```python
from build123d import *

# Parameters (mm, degrees)
BOSS_EXTRUDE2_DEPTH = 10
CUT_EXTRUDE9_DEPTH  = 3
BOSS_EXTRUDE3_DEPTH = 25
CUT_EXTRUDE11_DEPTH = 15


with BuildPart() as part:
    # Sketch1 → Boss-Extrude2 (new body)
    with BuildSketch(Plane(origin=(0, 0, 0), x_dir=(0, 0, -1), z_dir=(1, 0, 0))):
        Polygon((0, 0), (2, 0), (2, 9.1), (6.2, 13.3), (30, 13.3), (30, 15.3), (0, 15.3), align=None)
    extrude(amount=BOSS_EXTRUDE2_DEPTH)

    # Sketch2 → Cut-Extrude9 (cut)
    with BuildSketch(Plane(origin=(0, 15.3, 0), x_dir=(1, 0, 0), z_dir=(0, 1, 0))):
        with BuildLine():
            ThreePointArc((7, 15), (5, 17), (3, 15))
            Line((3, 15), (7, 15))
        make_face()
        with BuildLine():
            Line((7, 15), (3, 15))
            ThreePointArc((3, 15), (5, 13), (7, 15))
        make_face()
    extrude(amount=-CUT_EXTRUDE9_DEPTH, mode=Mode.SUBTRACT)

    # Sketch1<14> → Boss-Extrude3 (add)
    with BuildSketch(Plane(origin=(0, 0, 0), x_dir=(0, 0, -1), z_dir=(1, 0, 0))):
        Polygon((0, 7.6), (0, 0), (2, 0), (2, 9.1), (6.2, 13.3), (6.2, 15.3), (0, 15.3), (0, 12.4), (-1.8, 12.4), (-1.8, 15.25), (-4.55, 12.5), (-4.55, 7.671680622), (-1.8, 4.921680622), (-1.8, 7.6), align=None)
    extrude(amount=-BOSS_EXTRUDE3_DEPTH)

    # Sketch1<18> → Cut-Extrude11 (cut)
    with BuildSketch(Plane(origin=(0, 0, 0), x_dir=(0, 0, -1), z_dir=(1, 0, 0))):
        Polygon((-1.8, 7.6), (0, 7.6), (0, 12.4), (-1.8, 12.4), (-1.8, 15.25), (-4.55, 12.5), (-4.55, 7.671680622), (-1.8, 4.921680622), align=None)
    extrude(amount=-CUT_EXTRUDE11_DEPTH, mode=Mode.SUBTRACT)


solid = part.part
```
Input: part model. Units: mm. Frame: model coordinates. A direction names the side the tool comes from. Coordinates: 2 decimals unless noted, no trailing zeros. Loops run counter-clockwise (first coordinate to the right, second up) from the corner with the lowest first, then second, coordinate; pieces in that order, holes last. Notation, with made-up numbers: M 52,15.5 L 107,15.5 A7 ccw 107,24.5 Z; hole C 23.25,83 d5. An arc over 180 degrees is marked long. Answer in a Markdown table with one row per item.
1. Material intervals for line 1 (Z direction, x = 5, y = 14.05); line 2 (Z direction, x = -11.5, y = 6); line 3 (Z direction, x = -19.5, y = 6.25), sorted ascending.
Response:
| item | result |
|---|---|
| line 1 | z = -30 to -17, -13 to 0 |
| line 2 | z = -2 to 0 |
| line 3 | z = -2 to 0, 1.8 to 3.13 |
2. Draft query along Z for faces 1 (the flat face through (-12, 14, -6.2)), 2 (the flat face through (5, 13.3, -18)), 3 (the flat face through (-20, 12.4, 1)). Return one class per face: pulls with the +Z half, pulls with the -Z half, needs draft (parallel to the pull), parting line crosses it, or undercut.
Response:
| item | result |
|---|---|
| face 1 | pulls with the -Z half |
| face 2 | needs draft |
| face 3 | undercut |
3. First-contact query: pin 1 (3 mm diameter, centred on x = 5, z = -15, fed in from -Y); pin 2 (1.4 mm diameter, centred on x = -21, y = 13.5, fed in from -Z); pin 3 (4.5 mm diameter, centred on x = -16, y = 3, fed in from -Z); pin 4 (5 mm diameter, centred on x = -4.5, y = 4.5, fed in from +Z). Flat tips, straight axial feed; report the tip coordinate or a pass-through.
Response:
| item | result |
|---|---|
| pin 1 | passes through |
| pin 2 | stops at z = -6.2 |
| pin 3 | stops at z = -2 |
| pin 4 | stops at z = 0 |
4. Section C-C, the plane x = -5. Output: boundary loops of the cut face in (y, z), then the cut area to 3 significant figures.
Response:
| item | result |
|---|---|
| outline | M 0,-2 L 9.1,-2 L 13.3,-6.2 L 15.3,-6.2 L 15.3,0 L 0,0 Z |
| area | 47.8 mm2 |
5. Reachability of faces 4 (the flat face through (0, 14, -18)), 5 (the flat face through (-20, 14, 1.8)), 6 (the flat face through (-15, 10, 2)) from +Z, -Z, +X, -X, +Y, -Y: full face, straight path, thin tool, end or side. Return the list, or none.
Response:
| item | result |
|---|---|
| face 4 | -Z, -X, +Y, -Y |
| face 5 | +X, -X, +Y |
| face 6 | +Z, +X, +Y, -Y |
6. Section D-D, the plane z = -4. Output: boundary loops of the cut face in (x, y).
Response:
| item | result |
|---|---|
| outline | M -25,11.1 L 10,11.1 L 10,15.3 L -25,15.3 Z |
7. Section B-B, the plane x = 5. Output: boundary loops of the cut face in (y, z), then the cut area to 3 significant figures.
Response:
| item | result |
|---|---|
| outline | M 0,-2 L 9.1,-2 L 13.3,-6.2 L 13.3,-13 L 15.3,-13 L 15.3,0 L 0,0 Z; M 13.3,-30 L 15.3,-30 L 15.3,-17 L 13.3,-17 Z |
| area | 87.4 mm2 |
8. Section A-A, the plane z = -15. Output: boundary loops of the cut face in (x, y), then the cut area to 3 significant figures.
Response:
| item | result |
|---|---|
| outline | M 0,13.3 L 3,13.3 L 3,15.3 L 0,15.3 Z; M 7,13.3 L 10,13.3 L 10,15.3 L 7,15.3 Z |
| area | 12.0 mm2 |
